Check sheet for the modelled part. Datum: model origin and axes. Units: mm. Round coordinates to 2 decimals unless told otherwise and drop trailing zeros. Write each loop counter-clockwise with the first axis right and the second up, starting at its lowest first coordinate (ties: lowest second). Pieces come first, ordered by that corner, then holes.
Item 1: Release check for a two-part mould opening along X. For faces 1 (the flat face through (34.182, 150, -27)), 2 (the cylindrical face through (-42.4, 301.6, -27.4)), 3 (the cylindrical face through (-40.311, 108.087, -27.382)), 4 (the flat face through (-8, 150, -24.252)) record: +X half, -X half, draft (parallel to the pull), parting line (faces both ways), or undercut.
Item 2: Cross-section at A-A on y = 105.41. Enter the section's corners in (x, z), plus the area to 3 significant figures.
Item 3: Go/stop test with a flat-tipped pin: pin 1 Ø10 at (x, y) = (29.1, 105.41) entering from -Z. Record where the tip stops, or that it passes through.
Item 4: Material ranges on line 1 (X direction, y = 201.93, z = -28.5); line 2 (Y direction, x = 29, z = -29.25); line 3 (Y direction, x = 30.5, z = -25.5), recorded low to high.
from build123d import *

# Parameters (mm, degrees)
SKETCH1_W                 = 82.55
SKETCH1_H                 = 6.35
BOSS_EXTRUDE1_DEPTH       = 304.8
SKETCH2_R                 = 3.175
CUT_EXTRUDE1_DEPTH        = 152.4
LPATTERN1_COUNT           = 4
LPATTERN1_PITCH           = 96.52
LPATTERN2_COUNT           = 2
LPATTERN2_PITCH           = 71.12
LPATTERN2_COPY_1_SKETCH_R = 3.175
LPATTERN2_COPY_1_DEPTH    = 152.4
LPATTERN2_COPY_2_SKETCH_R = 3.175
LPATTERN2_COPY_2_DEPTH    = 152.4
LPATTERN2_COPY_3_SKETCH_R = 3.175
LPATTERN2_COPY_3_DEPTH    = 152.4


with BuildPart() as part:
    # Sketch1 → Boss-Extrude1 (new body)
    with BuildSketch(Plane(origin=(0, 0, 0), x_dir=(1, 0, 0), z_dir=(0, 1, 0))):
        with Locations((-7.093085106, 27.426595745)):
            Rectangle(SKETCH1_W, SKETCH1_H)
    extrude(amount=BOSS_EXTRUDE1_DEPTH)

    # Sketch2 → Cut-Extrude1 (cut)
    with BuildSketch(Plane.XY.offset(-24.251595745)):
        with Locations((-42.018085106, 298.45)):
            Circle(SKETCH2_R)
    cut_extrude1 = extrude(amount=-CUT_EXTRUDE1_DEPTH, mode=Mode.SUBTRACT)

    # LPattern1: Cut-Extrude1 ×4
    with Locations(*[(0, -i * LPATTERN1_PITCH, 0) for i in range(1, LPATTERN1_COUNT)]):
        add(cut_extrude1, mode=Mode.SUBTRACT)

    # LPattern2: Cut-Extrude1 ×2
    with Locations(*[(i * LPATTERN2_PITCH, 0, 0) for i in range(1, LPATTERN2_COUNT)]):
        add(cut_extrude1, mode=Mode.SUBTRACT)

    # LPattern2 copy 1 sketch → LPattern2 copy 1 (cut)
    with BuildSketch(Plane(origin=(71.12, -96.52, -24.251595745), x_dir=(1, 0, 0), z_dir=(0, 0, 1))):
        with Locations((-42.018085106, 298.45)):
            Circle(LPATTERN2_COPY_1_SKETCH_R)
    extrude(amount=-LPATTERN2_COPY_1_DEPTH, mode=Mode.SUBTRACT)

    # LPattern2 copy 2 sketch → LPattern2 copy 2 (cut)
    with BuildSketch(Plane(origin=(71.12, -193.04, -24.251595745), x_dir=(1, 0, 0), z_dir=(0, 0, 1))):
        with Locations((-42.018085106, 298.45)):
            Circle(LPATTERN2_COPY_2_SKETCH_R)
    extrude(amount=-LPATTERN2_COPY_2_DEPTH, mode=Mode.SUBTRACT)

    # LPattern2 copy 3 sketch → LPattern2 copy 3 (cut)
    with BuildSketch(Plane(origin=(71.12, -289.56, -24.251595745), x_dir=(1, 0, 0), z_dir=(0, 0, 1))):
        with Locations((-42.018085106, 298.45)):
            Circle(LPATTERN2_COPY_3_SKETCH_R)
    extrude(amount=-LPATTERN2_COPY_3_DEPTH, mode=Mode.SUBTRACT)


solid = part.part
Response values:
1. face 1: +X half
1. face 2: undercut
1. face 3: undercut
1. face 4: draft
2. outline: (-48.37, -30.6) - (-45.19, -30.6) - (-45.19, -24.25) - (-48.37, -24.25) - close; (-38.84, -30.6) - (25.93, -30.6) - (25.93, -24.25) - (-38.84, -24.25) - close; (32.28, -30.6) - (34.18, -30.6) - (34.18, -24.25) - (32.28, -24.25) - close
2. area: 444 mm2
3. pin 1: stops at z = -30.6
4. line 1: x = -48.37 to -45.19, -38.84 to 25.93, 32.28 to 34.18
4. line 2: y = 0 to 5.72, 12.06 to 102.24, 108.58 to 198.76, 205.1 to 295.28, 301.62 to 304.8
4. line 3: y = 0 to 6.04, 11.74 to 102.56, 108.26 to 199.08, 204.78 to 295.6, 301.3 to 304.8
